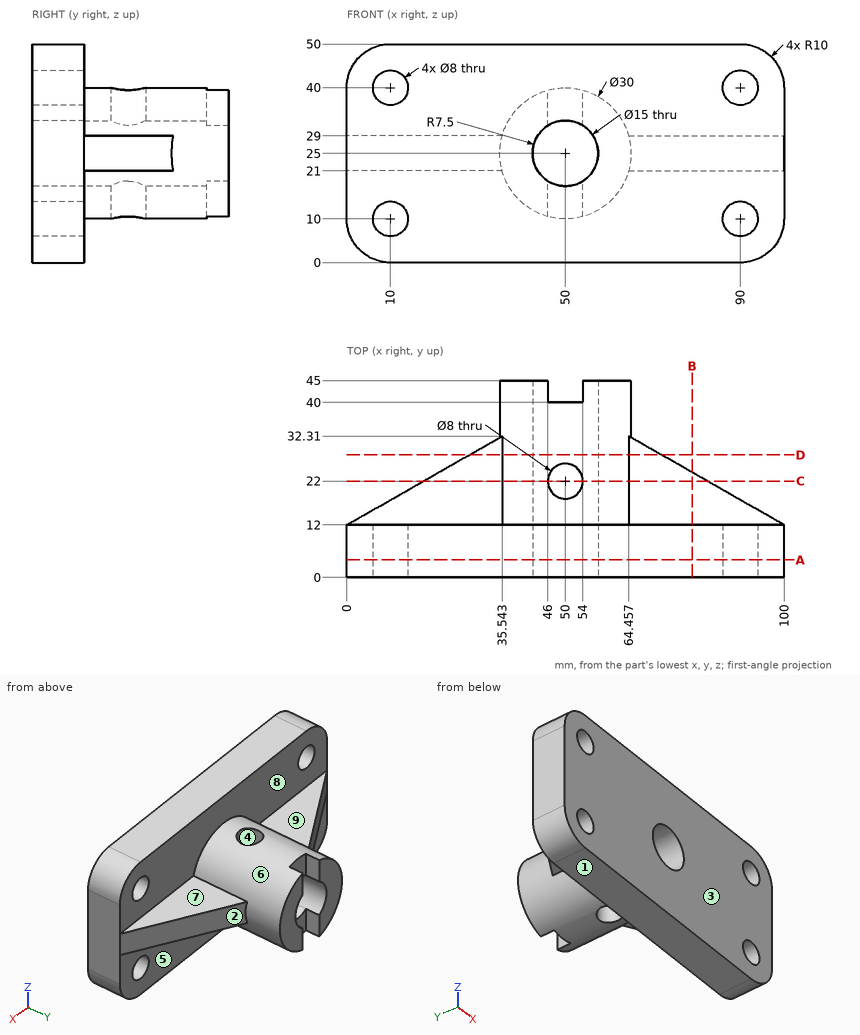
Geometry: see drawing. Coordinates: mm, zero at the bounding-box minimum. A direction names the side the tool comes from. Coordinates: 2 decimals unless noted, no trailing zeros. Loops run counter-clockwise (first coordinate to the right, second up) from the corner with the lowest first, then second, coordinate; pieces in that order, holes last. Notation, with made-up numbers: (10, 46) -> (22, 46) arc R30 cw to (22, 82) -> close; hole circle Ø11 at (-36.5, 82). An arc over 180 degrees is marked (long way). Use a Markdown table: item, result.
1) Material intervals for line 1 along X through (y, z) = (6.5, 10); line 2 along Y through (x, z) = (50, 15); line 3 along Z through (x, y) = (50, 6), sorted ascending. Write a range as from..to.
Results found:
| item | result |
|---|---|
| line 1 | x = 0..6, 14..86, 94..100 |
| line 2 | y = 0..18, 26..40 |
| line 3 | z = 0..17.5, 32.5..50 |
2) Cut plane D-D (y = 28). Return the cut outline in (x, z) (1 decimal).
Results found:
| item | result |
|---|---|
| outline | (28, 21) -> (35.5, 21) arc R15 ccw to (64.5, 21) -> (72, 21) -> (72, 29) -> (64.5, 29) arc R15 ccw to (35.5, 29) -> (28, 29) -> close; hole circle Ø15 at (50, 25) |
3) Access query for the marked faces 5, 6, 7, 8 and 9. Directions: +Z, -Z, +X, -X, +Y, -Y. A direction counts if a zero-diameter tool reaches every point of the face in a straight line with its end or side. Return the directions, or none.
Results found:
| item | result |
|---|---|
| face 5 | -Z, +Y |
| face 6 | +Y |
| face 7 | +Z, +X, +Y |
| face 8 | +Z, +Y |
| face 9 | +Z, -X, +Y |
4) Pull-direction query (Y, two-part tool) for the marked faces 1, 2, 3 and 4; classes: released by +Y, released by -Y, zero draft, split by the parting line, or undercut.
Results found:
| item | result |
|---|---|
| face 1 | zero draft |
| face 2 | released by +Y |
| face 3 | released by -Y |
| face 4 | undercut |
5) Cut plane C-C (y = 22). Return the cut outline in (x, z) (1 decimal).
Results found:
| item | result |
|---|---|
| outline | (17.5, 21) -> (35.5, 21) arc R15 ccw to (46, 10.5) -> (46, 18.7) arc R7.5 cw to (46, 31.3) -> (46, 39.5) arc R15 ccw to (35.5, 29) -> (17.5, 29) -> close; (54, 10.5) arc R15 ccw to (64.5, 21) -> (82.5, 21) -> (82.5, 29) -> (64.5, 29) arc R15 ccw to (54, 39.5) -> (54, 31.3) arc R7.5 cw to (54, 18.7) -> close |
6) Cut plane A-A (y = 4). Return the cut outline in (x, z) (1 decimal), then the cut area to 3 significant figures.
Results found:
| item | result |
|---|---|
| outline | (0, 10) arc R10 ccw to (10, 0) -> (90, 0) arc R10 ccw to (100, 10) -> (100, 40) arc R10 ccw to (90, 50) -> (10, 50) arc R10 ccw to (0, 40) -> close; hole circle Ø8 at (10, 10); hole circle Ø8 at (10, 40); hole circle Ø15 at (50, 25); hole circle Ø8 at (90, 10); hole circle Ø8 at (90, 40) |
| area | 4,540 mm2 |
7) Cut plane B-B (x = 79). Return the cut outline in (y, z), then the cut area to 3 significant figures.
Results found:
| item | result |
|---|---|
| outline | (0, 0) -> (12, 0) -> (12, 21) -> (24, 21) -> (24, 29) -> (12, 29) -> (12, 50) -> (0, 50) -> close |
| area | 696 mm2 |
8) Contact query for flat-ended pins moving along their axis: pin 1 (6 mm diameter, centred on x = 12.5, y = 25, fed in from -Z); pin 2 (16 mm diameter, centred on x = 85, y = 21, fed in from -Z); pin 3 (2 mm diameter, centred on y = 30.5, z = 32.5, fed in from +X); pin 4 (4 mm diameter, centred on y = 43.5, z = 37, fed in from -X). Output: stop coordinate, or through.
Results found:
| item | result |
|---|---|
| pin 1 | passes through |
| pin 2 | stops at z = 21 |
| pin 3 | stops at x = 63.52 |
| pin 4 | stops at x = 38.82 |
